from build123d import *

# Parameters (mm, degrees)
ESQUISSE1_W             = 100
ESQUISSE1_H             = 80
BOSS_EXTRU_1_DEPTH      = 2
ESQUISSE2_W             = 100
ESQUISSE2_H             = 80
ESQUISSE2_W_2           = 96
ESQUISSE2_H_2           = 76
ESQUISSE2_R             = 2
BOSS_EXTRU_2_DEPTH      = 3
ESQUISSE3_R             = 0.75
ENL_V_MAT_EXTRU_1_DEPTH = 5
ESQUISSE4_R             = 1.5
ENL_V_MAT_EXTRU_2_DEPTH = 5
ESQUISSE5_W             = 98
ESQUISSE5_H             = 78
ESQUISSE5_W_2           = 96
ESQUISSE5_H_2           = 76
BOSS_EXTRU_3_DEPTH      = 2
ESQUISSE6_W             = 20
ESQUISSE6_H             = 5
BOSS_EXTRU_4_DEPTH      = 3
ESQUISSE7_W             = 1
ESQUISSE7_H             = 5
BOSS_EXTRU_5_DEPTH      = 2
ESQUISSE8_W             = 18
ESQUISSE8_H             = 2
ENL_V_MAT_EXTRU_3_DEPTH = 2


with BuildPart() as part:
    # Esquisse1 → Boss.-Extru.1 (new body)
    with BuildSketch(Plane(origin=(0, 0, 0), x_dir=(1, 0, 0), z_dir=(0, 1, 0))):
        Rectangle(ESQUISSE1_W, ESQUISSE1_H)
    extrude(amount=BOSS_EXTRU_1_DEPTH)

    # Esquisse2 → Boss.-Extru.2 (add)
    with BuildSketch(Plane(origin=(0, 2, 0), x_dir=(1, 0, 0), z_dir=(0, 1, 0))):
        Rectangle(ESQUISSE2_W, ESQUISSE2_H)
        Rectangle(ESQUISSE2_W_2, ESQUISSE2_H_2, mode=Mode.SUBTRACT)
        with Locations((38, -34)):
            Circle(ESQUISSE2_R)
        with Locations((38, 2)):
            Circle(ESQUISSE2_R)
        with Locations((-38, -34)):
            Circle(ESQUISSE2_R)
        with Locations((-38, 2)):
            Circle(ESQUISSE2_R)
    extrude(amount=BOSS_EXTRU_2_DEPTH)

    # Esquisse3 → Enlèv. mat.-Extru.1 (cut)
    with BuildSketch(Plane(origin=(0, 5, 0), x_dir=(1, 0, 0), z_dir=(0, 1, 0))):
        with Locations((-38, 2)):
            Circle(ESQUISSE3_R)
        with Locations((-38, -34)):
            Circle(ESQUISSE3_R)
        with Locations((38, 2)):
            Circle(ESQUISSE3_R)
        with Locations((38, -34)):
            Circle(ESQUISSE3_R)
    extrude(amount=-ENL_V_MAT_EXTRU_1_DEPTH, mode=Mode.SUBTRACT)

    # Esquisse4 → Enlèv. mat.-Extru.2 (cut)
    with BuildSketch(Plane(origin=(0, 2, 0), x_dir=(1, 0, 0), z_dir=(0, 1, 0))):
        with Locations((-44, 34)):
            Circle(ESQUISSE4_R)
        with Locations((44, 34)):
            Circle(ESQUISSE4_R)
        with Locations((44, -34)):
            Circle(ESQUISSE4_R)
        with Locations((-44, -34)):
            Circle(ESQUISSE4_R)
    extrude(amount=-ENL_V_MAT_EXTRU_2_DEPTH, mode=Mode.SUBTRACT)

    # Esquisse5 → Boss.-Extru.3 (add)
    with BuildSketch(Plane(origin=(0, 5, 0), x_dir=(1, 0, 0), z_dir=(0, 1, 0))):
        Rectangle(ESQUISSE5_W, ESQUISSE5_H)
        Rectangle(ESQUISSE5_W_2, ESQUISSE5_H_2, mode=Mode.SUBTRACT)
    extrude(amount=BOSS_EXTRU_3_DEPTH)

    # Esquisse6 → Boss.-Extru.4 (add)
    with BuildSketch(Plane(origin=(0, 2, 0), x_dir=(1, 0, 0), z_dir=(0, 1, 0))):
        with Locations((30, 35.5)):
            Rectangle(ESQUISSE6_W, ESQUISSE6_H)
    extrude(amount=BOSS_EXTRU_4_DEPTH)

    # Esquisse7 → Boss.-Extru.5 (add)
    with BuildSketch(Plane(origin=(0, 5, 0), x_dir=(1, 0, 0), z_dir=(0, 1, 0))):
        with Locations((20.5, 35.5)):
            Rectangle(ESQUISSE7_W, ESQUISSE7_H)
        with Locations((39.5, 35.5)):
            Rectangle(ESQUISSE7_W, ESQUISSE7_H)
    extrude(amount=BOSS_EXTRU_5_DEPTH)

    # Esquisse8 → Enlèv. mat.-Extru.3 (cut)
    with BuildSketch(Plane.XY.offset(-38)):
        with Locations((30, 6)):
            Rectangle(ESQUISSE8_W, ESQUISSE8_H)
    extrude(amount=-ENL_V_MAT_EXTRU_3_DEPTH, mode=Mode.SUBTRACT)


solid = part.part
Build history of the part. All positions in model axes, mm. A direction names the side the tool comes from. Give positions to 0.01 mm unless a question says otherwise; leave off trailing zeros. Order: outer loops, then holes, each group sorted by start corner. A loop starts at its lowest first (then second) coordinate and runs counter-clockwise, first axis right, second up. Notation, with made-up numbers: M -10,19 L 22,19 A12 cw 22,38 Z; hole C -12,46.25 d3. An arc over 180 degrees is marked long. Use one line per item in the form item = value.
1) Saw through at B-B (x = 44). Give the cut face in (y, z).
Calculated:
outline = M 0,-40 L 5,-40 L 5,-39 L 7,-39 L 7,-38 L 2,-38 L 2,-35.5 L 0,-35.5 Z; M 0,-32.5 L 2,-32.5 L 2,32.5 L 0,32.5 Z; M 0,35.5 L 2,35.5 L 2,38 L 7,38 L 7,39 L 5,39 L 5,40 L 0,40 Z
2) Saw through at C-C (z = 21). Give the cut face in (x, y).
Calculated:
outline = M -50,0 L 50,0 L 50,5 L 49,5 L 49,7 L 48,7 L 48,2 L -48,2 L -48,7 L -49,7 L -49,5 L -50,5 Z
3) Drop flat-ended pins along their axis: pin 1 (5 mm diameter, centred on x = -33, z = 18, fed in from +Y); pin 2 (0.9 mm diameter, centred on x = 38, z = -2, fed in from -Y); pin 3 (0.6 mm diameter, centred on y = 5.5, z = -36, fed in from -X); pin 4 (3 mm diameter, centred on x = 39, z = -2.5, fed in from +Y). Give the stop position or say it passes through.
Calculated:
pin_1 = 2
pin_2 = through
pin_3 = -49
pin_4 = 5
4) Tool access for faces 5 (the face through (49, 6, 1)), 6 (the face through (50, 2, 1)), 7 (the face through (21, 6, -36)), 8 (the face through (38, 5, 35)), 9 (the face through (-49, 6, 1)): list every direction of +Z, -Z, +X, -X, +Y, -Y with a clear straight run to the whole face (end or side of a thin tool).
Calculated:
face_5 = +Z, -Z, +X, +Y
face_6 = +Z, -Z, +X, +Y, -Y
face_7 = -Z, +Y
face_8 = +Y
face_9 = +Z, -Z, -X, +Y
5) Probe probe 1 along Z at (x, y) = (-44, 0.6); probe 2 along X at (y, z) = (1.1, 34); probe 3 along X at (y, z) = (3.25, -7). List the from-to ranges inside material, lowest first.
Calculated:
probe_1 = -40 to -35.5, -32.5 to 32.5, 35.5 to 40
probe_2 = -50 to -45.5, -42.5 to -38.75, -37.25 to 37.25, 38.75 to 42.5, 45.5 to 50
probe_3 = -50 to -48, 48 to 50
6) Saw through at D-D (x = 27). Give the cut face in (y, z).
Calculated:
outline = M 0,-40 L 5,-40 L 5,-33 L 2,-33 L 2,38 L 7,38 L 7,39 L 5,39 L 5,40 L 0,40 Z
7) Saw through at A-A (y = 3.25). State how many separate pieces and enclosed holes the cut face has, plus the area to 3 significant figures.
Calculated:
separate_pieces = 5
enclosed_holes = 5
area = 847 mm2
8) Two-plate mould, pull along Z, no slides. Class faces 1 (the face through (-50, 2, 1)), 2 (the face through (-38, 5, -1)), 3 (the face through (44, 6, -39)), 4 (the face through (-48, 4, 1)): released by +Z, released by -Z, zero draft, split by the parting line, or undercut.
Calculated:
face_1 = zero draft
face_2 = undercut
face_3 = released by -Z
face_4 = undercut
